```python
from build123d import *

# Parameters (mm, degrees)
F0_R     = 1.5
F1_DEPTH = 1.6


with BuildPart() as f1:
    # F0 (on Top) → F1 (new body)
    with BuildSketch(Plane.XY):
        with BuildLine():
            ThreePointArc((17.5, 29.5), (16.62132, 31.62132), (14.5, 32.5))
            Line((14.5, 32.5), (-14.5, 32.5))
            ThreePointArc((-14.5, 32.5), (-16.62132, 31.62132), (-17.5, 29.5))
            Line((-17.5, 29.5), (-17.5, -29.5))
            ThreePointArc((-17.5, -29.5), (-16.62132, -31.62132), (-14.5, -32.5))
            Line((-14.5, -32.5), (14.5, -32.5))
            ThreePointArc((14.5, -32.5), (16.62132, -31.62132), (17.5, -29.5))
            Line((17.5, -29.5), (17.5, 29.5))
        make_face()
        with Locations((-14, -29)):
            Circle(F0_R, mode=Mode.SUBTRACT)
        with Locations((14, -29)):
            Circle(F0_R, mode=Mode.SUBTRACT)
        with Locations((-14, 29)):
            Circle(F0_R, mode=Mode.SUBTRACT)
        with Locations((14, 29)):
            Circle(F0_R, mode=Mode.SUBTRACT)
    extrude(amount=-F1_DEPTH)


solid = f1.part
```
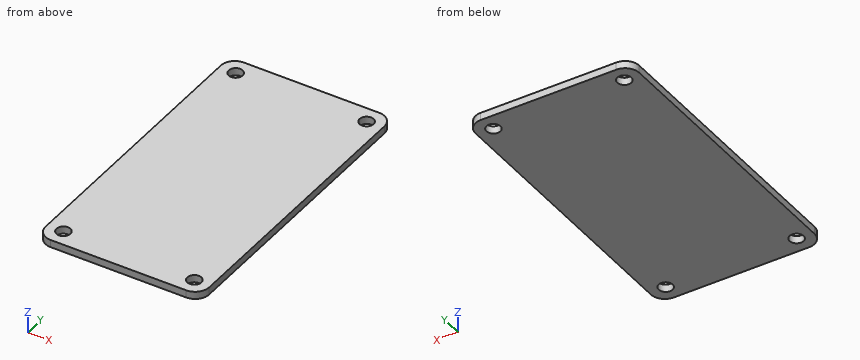
Here's how the part is built. I have some questions about the finished solid (model axes, mm). Round coordinates to 2 decimals unless told otherwise and drop trailing zeros. Loops run counter-clockwise (first coordinate to the right, second up) from the corner with the lowest first, then second, coordinate; pieces in that order, holes last.
1. Will these pins go through, and if not, where does the flat tip stop? pin 1 (5 mm diameter, centred on x = 14, y = -29, fed in from -Z); pin 2 (2.5 mm diameter, centred on x = 14, y = 29, fed in from +Z).
Answers:
pin 1: stops at z = -1.6
pin 2: passes through
2. If I drill on probe 1 along Y at (x, z) = (14, -0.6); probe 2 along Y at (x, z) = (-13.5, -0.3), over which ranges is the centre line in solid material (lowest first)?
Answers:
probe 1: y = -32.5 to -30.5, -27.5 to 27.5, 30.5 to 32.5
probe 2: y = -32.5 to -30.41, -27.59 to 27.59, 30.41 to 32.5
3. Suppose I cut it at A-A, the plane z = -0.8. Please give me the cut outline in (x, y).
Answers:
outline: (-17.5, -29.5) arc R3 ccw to (-14.5, -32.5) - (14.5, -32.5) arc R3 ccw to (17.5, -29.5) - (17.5, 29.5) arc R3 ccw to (14.5, 32.5) - (-14.5, 32.5) arc R3 ccw to (-17.5, 29.5) - close; hole circle Ø3 at (-14, -29); hole circle Ø3 at (-14, 29); hole circle Ø3 at (14, -29); hole circle Ø3 at (14, 29)
